Work out the finished part from the listing and answer in its coordinate system (mm). A direction names the side the tool comes from. Coordinates: 2 decimals unless noted, no trailing zeros. Loops run counter-clockwise (first coordinate to the right, second up) from the corner with the lowest first, then second, coordinate; pieces in that order, holes last. Notation, with made-up numbers: (74.5, 79) - (108.5, 79) arc R23 ccw to (108.5, 98) - close; hole circle Ø5 at (15, -17). An arc over 180 degrees is marked (long way). Write each question's results on one line, items separated by ' | '. Start each with the question number.
Item 1: Each of these flat-tipped pins is pushed along its axis until it touches: pin 1 Ø0.5 at (x, y) = (0, -2) entering from +Z; pin 2 Ø0.5 at (x, y) = (0.5, -2) entering from -Z; pin 3 Ø1.4 at (y, z) = (-2, -6) entering from +X; pin 4 Ø4 at (x, z) = (2, -5.5) entering from -Y. Where does it stop, or does it pass through?
Item 2: Section A-A, the plane x = 0 is taken. Write down the section's boundary in (y, z).
Item 3: Consider probe 1 along Z at (x, y) = (0, -0.45); probe 2 along Y at (x, z) = (3, -8.25); probe 3 along Z at (x, y) = (-3, 3.5). Determine where each line is inside the solid, lowest interval first. Write a range as [from, to].
Item 4: Section C-C, the plane x = -2.25 is taken. Write down the section's boundary in (y, z).
Item 5: For a pull along Z with two mould halves and no side action, classify faces 5 (the face through (0.86, -0.44, 0.27)), 6 (the face through (0, 8, -11.3)), 7 (the face through (-1.35, -2, -6)), 8 (the face through (0, 8, -8)) as +Z half, -Z half, draft (parallel to the pull), parting line (faces both ways), or undercut.
Item 6: A tool of negligible diameter and unlimited length cuts with its end or side. For faces 1 (the face through (1.35, -2, -6)), 2 (the face through (0, 0, -3)), 3 (the face through (0, -2, -4.65)), 4 (the face through (0, -2, -8)), from which of +Z, -Z, +X, -X, +Y, -Y can it reach the whole face along a straight path? Write none if from no direction.
Item 7: Section B-B, the plane z = 0 is taken. Write down the section's boundary in (x, y) (3 decimals).
Item 8: Section D-D, the plane y = 8 is taken. Write down the section's boundary in (x, z) (3 decimals), plus the area to 3 significant figures.
from build123d import *

# Parameters (mm, degrees)
F0_W     = 7.65
F0_H     = 12.6
F0_R     = 0.9
F1_DEPTH = 0.9
F2_W     = 7.65
F2_H     = 3.3
F3_DEPTH = 17
F4_W     = 2.7
F4_H     = 3.35
F5_DEPTH = 1.7


with BuildPart() as f1:
    # F0 (on Front) → F1 (new body)
    with BuildSketch(Plane.XZ):
        with Locations((0, -4.5)):
            Rectangle(F0_W, F0_H)
        Circle(F0_R, mode=Mode.SUBTRACT)
    extrude(amount=F1_DEPTH)

    # F2 (on face) → F3 (join)
    with BuildSketch(Plane(origin=(0, 0, 0), x_dir=(-1, 0, 0), z_dir=(0, 1, 0))):
        with Locations((0, -9.65)):
            Rectangle(F2_W, F2_H)
    extrude(amount=F3_DEPTH)

    # F4 (on face) → F5 (join)
    with BuildSketch(Plane.XZ.offset(0.9)):
        with Locations((0, -6.325)):
            Rectangle(F4_W, F4_H)
    extrude(amount=F5_DEPTH)


solid = f1.part
Answer key:
1) pin 1: stops at z = -4.65 | pin 2: stops at z = -8 | pin 3: stops at x = 1.35 | pin 4: stops at y = -2.6
2) outline: (-2.6, -8) - (-0.9, -8) - (-0.9, -10.8) - (0, -10.8) - (0, -11.3) - (17, -11.3) - (17, -8) - (0, -8) - (0, -0.9) - (-0.9, -0.9) - (-0.9, -4.65) - (-2.6, -4.65) - close; (-0.9, 0.9) - (0, 0.9) - (0, 1.8) - (-0.9, 1.8) - close
3) probe 1: z = [-10.8, -0.9], [0.9, 1.8] | probe 2: y = [-0.9, 17] | probe 3: z = [-11.3, -8]
4) outline: (-0.9, -10.8) - (0, -10.8) - (0, -11.3) - (17, -11.3) - (17, -8) - (0, -8) - (0, 1.8) - (-0.9, 1.8) - close
5) face 5: undercut | face 6: -Z half | face 7: draft | face 8: +Z half
6) face 1: +Z, -Z, +X, -Y | face 2: +Z, +X, -X, +Y | face 3: +Z, +X, -X, -Y | face 4: -Z, +X, -X, -Y
7) outline: (-3.825, -0.9) - (-0.9, -0.9) - (-0.9, 0) - (-3.825, 0) - close; (0.9, -0.9) - (3.825, -0.9) - (3.825, 0) - (0.9, 0) - close
8) outline: (-3.825, -11.3) - (3.825, -11.3) - (3.825, -8) - (-3.825, -8) - close | area: 25.2 mm^2
